CAD build for the part. Positions are in the model's coordinates, mm. A direction names the side the tool comes from. Coordinates: 2 decimals unless noted, no trailing zeros. Loops run counter-clockwise (first coordinate to the right, second up) from the corner with the lowest first, then second, coordinate; pieces in that order, holes last.
1) Wall check: line 1 along Z through (x, y) = (1, 22); line 2 along Z through (x, y) = (-11, 1); line 3 along X through (y, z) = (7, 38). Give the ranges that are in metal, low to high.
2) Saw through at D-D, the plane y = -0.5. Write the cut outline in (x, z).
3) Saw through at A-A, the plane y = 7. Write the cut outline in (x, z), and give its area (3 significant figures).
4) Which spindle directions (+Z, -Z, +X, -X, +Y, -Y) get a long thin tool onto all of the face, cutting with end or side? Do faces 1 (the flat face through (-10, 11, 30)), 2 (the flat face through (-4, -17.872, 8)). Say none if no direction does.
5) Pin check, flat tips, straight feed: pin 1 Ø9 at (x, y) = (1, 18) entering from +Z; pin 2 Ø12 at (y, z) = (12, 30.5) entering from -X; pin 3 Ø3 at (x, z) = (-37.5, 9.5) entering from -Y. Stop position of each tip, or through.
6) Saw through at B-B, the plane x = -9. Write the cut outline in (y, z).
```python
from build123d import *

# Parameters (mm, degrees)
F1_DEPTH = 10
F2_DEPTH = 30
F3_DEPTH = 40


with BuildPart() as f1:
    # F0 (on Top) → F1 (new body)
    with BuildSketch(Plane.XY):
        Polygon((21.850749, -17.87234), (9.574469, 38.723405), (0, 38.723405), (-7.665832, -17.87234), align=None)
    extrude(amount=F1_DEPTH)

    # F0 (on Top) → F2 (join)
    with BuildSketch(Plane.XY):
        Polygon((-7.665832, -17.87234), (0, 38.723405), (-10, 38.723405), (-20.425531, -17.87234), align=None)
    extrude(amount=F2_DEPTH)

    # F0 (on Top) → F3 (join)
    with BuildSketch(Plane.XY):
        with BuildLine():
            Line((-20.425531, -17.87234), (-10, 38.723405))
            Line((-10, 38.723405), (-20.425531, 38.723405))
            ThreePointArc((-20.425531, 38.723405), (-47.679565, 10.425532), (-20.425531, -17.87234))
        make_face()
    extrude(amount=F3_DEPTH)


solid = f1.part
```
Data:
1. line 1: z = 0 to 10
1. line 2: z = 0 to 30
1. line 3: x = -47.47 to -15.84
2. outline: (-45.49, 0) - (18.08, 0) - (18.08, 10) - (-5.31, 10) - (-5.31, 30) - (-17.23, 30) - (-17.23, 40) - (-45.49, 40) - close
3. outline: (-47.47, 0) - (16.46, 0) - (16.46, 10) - (-4.3, 10) - (-4.3, 30) - (-15.84, 30) - (-15.84, 40) - (-47.47, 40) - close
3. area: 1,820 mm2
4. face 1: +Z, +X, -Y
4. face 2: +Z, -Z, +X, -X, -Y
5. pin 1: stops at z = 30
5. pin 2: stops at x = -47.68
5. pin 3: stops at y = -12.49
6. outline: (-17.87, 0) - (38.72, 0) - (38.72, 30) - (-17.87, 30) - close
